Read the model definition and answer for the solid it produces. Units are mm, in the model's axes. A direction names the side the tool comes from. Coordinates: 2 decimals unless noted, no trailing zeros. Order: outer loops, then holes, each group sorted by start corner. A loop starts at its lowest first (then second) coordinate and runs counter-clockwise, first axis right, second up. Notation, with made-up numbers: M 71.25,-21.5 L 103.25,-21.5 A18 cw 103.25,-13.5 Z; hole C 14.25,58 d4. An arc over 180 degrees is marked long. One line per question, with ' | ' between items. Start each with the question number.
1) Consider probe 1 along Y at (x, z) = (90, 51.5); probe 2 along X at (y, z) = (28.5, 51). Determine where each line is inside the solid, lowest interval first.
2) Given P1, Ø7.5, axis at y = -16.5, z = 61.5, coming from the -X side; P2, Ø12.5, axis at x = -2, z = 69.5, coming from the +Y side, each flat-ended and moving along its own axis, determine where each tip first touches the part or whether it passes through.
3) A tool of negligible diameter and unlimited length cuts with its end or side. For faces 1 (the face through (7, -73.324, 64)), 2 (the face through (100, -71.3, 63.7)), 3 (the face through (5, 65.056, 64)), from which of +Z, -Z, +X, -X, +Y, -Y can it reach the whole face along a straight path? Write none if from no direction.
4) Find section A-A, the plane z = 61. Write down the section's boundary in (x, y), plus the area to 3 significant figures.
from build123d import *

# Parameters (mm, degrees)
F0_W     = 197.0488578081
F0_H     = 143.7139809132
F1_DEPTH = 76.2
F2_R     = 9.525
F4_DEPTH = 25.4


with BuildPart() as f1:
    # F0 (on Top) → F1 (new body, symmetric)
    with BuildSketch(Plane.XY):
        with Locations((6.136842072, -4.1339993477)):
            Rectangle(F0_W, F0_H)
    extrude(amount=F1_DEPTH, both=True)

    # F2
    f2_edges = [f1.edges().sort_by_distance(p)[0] for p in [
        (-92.387587, -75.99099, 0),
        (-92.387587, 67.722991, 0),
        (104.661271, 67.722991, 0),
        (104.661271, -75.99099, 0),
    ]]
    fillet(f2_edges, radius=F2_R)

    # F3 (on face) → F4 (cut)
    with BuildSketch(Plane.XY.offset(76.2)):
        with BuildLine():
            Line((95.1362709761, 67.7229911089), (-82.862586832, 67.7229911089))
            ThreePointArc((-82.862586832, 67.7229911089), (-89.5977789228, 64.9331831997), (-92.387586832, 58.1979911089))
            Line((-92.387586832, 58.1979911089), (-92.387586832, -66.4659898043))
            ThreePointArc((-92.387586832, -66.4659898043), (-89.5977789228, -73.2011818951), (-82.862586832, -75.9909898043))
            Line((-82.862586832, -75.9909898043), (95.1362709761, -75.9909898043))
            ThreePointArc((95.1362709761, -75.9909898043), (101.8714630669, -73.2011818951), (104.6612709761, -66.4659898043))
            Line((104.6612709761, -66.4659898043), (104.6612709761, 58.1979911089))
            ThreePointArc((104.6612709761, 58.1979911089), (101.8714630669, 64.9331831997), (95.1362709761, 67.7229911089))
        make_face()
        with BuildLine():
            ThreePointArc((-89.720586832, 58.1979911089), (-87.7119251374, 63.0473294143), (-82.862586832, 65.0559911089))
            Line((-82.862586832, 65.0559911089), (95.1362709761, 65.0559911089))
            ThreePointArc((95.1362709761, 65.0559911089), (99.9856092814, 63.0473294143), (101.9942709761, 58.1979911089))
            Line((101.9942709761, 58.1979911089), (101.9942709761, -66.4659898043))
            ThreePointArc((101.9942709761, -66.4659898043), (99.9856092814, -71.3153281096), (95.1362709761, -73.3239898043))
            Line((95.1362709761, -73.3239898043), (-82.862586832, -73.3239898043))
            ThreePointArc((-82.862586832, -73.3239898043), (-87.7119251374, -71.3153281096), (-89.720586832, -66.4659898043))
            Line((-89.720586832, -66.4659898043), (-89.720586832, 58.1979911089))
        make_face(mode=Mode.SUBTRACT)
    extrude(amount=-F4_DEPTH, mode=Mode.SUBTRACT)


solid = f1.part
Report:
1) probe 1: y = -73.32 to 65.06 | probe 2: x = -89.72 to 101.99
2) P1: stops at x = -89.72 | P2: stops at y = 65.06
3) face 1: +Z, +X, -X, -Y | face 2: +Z, +X, -Y | face 3: +Z, +X, -X, +Y
4) outline: M -89.72,-66.47 A6.86 ccw -82.86,-73.32 L 95.14,-73.32 A6.86 ccw 101.99,-66.47 L 101.99,58.2 A6.86 ccw 95.14,65.06 L -82.86,65.06 A6.86 ccw -89.72,58.2 Z | area: 26,500 mm^2
